For this review, take the finished solid that the model builds, in its own axes (mm). A direction names the side the tool comes from. Round coordinates to 2 decimals unless told otherwise and drop trailing zeros. Loops run counter-clockwise (first coordinate to the right, second up) from the corner with the lowest first, then second, coordinate; pieces in that order, holes last. Notation, with made-up numbers: (41, -8) -> (92, -8) arc R24 ccw to (92, 2) -> close; hole circle Ø2 at (65, 54). An arc over 180 degrees is marked (long way). Write each question's results on one line, items separated by ' | '.
```python
from build123d import *
from OCP.BRepFilletAPI import BRepFilletAPI_MakeChamfer

# Parameters (mm, degrees)
SKETCH1_W           = 60
SKETCH1_H           = 27
BOSS_EXTRUDE1_DEPTH = 6
SKETCH2_R           = 13.5
SKETCH2_R_2         = 8.5
BOSS_EXTRUDE2_DEPTH = 30
SKETCH3_W           = 60
SKETCH3_H           = 5
BOSS_EXTRUDE3_DEPTH = 30
CHAMFER1_SIZE       = 30
CHAMFER1_SIZE2      = 19.5
SKETCH5_R           = 2.5
CUT_EXTRUDE1_DEPTH  = 30
CHAMFER3_SIZE       = 1


with BuildPart() as part:
    # Sketch1 → Boss-Extrude1 (new body)
    with BuildSketch(Plane(origin=(0, 0, 0), x_dir=(1, 0, 0), z_dir=(0, 1, 0))):
        with Locations((-76.040322581, 2.721774194)):
            Rectangle(SKETCH1_W, SKETCH1_H)
    extrude(amount=BOSS_EXTRUDE1_DEPTH)

    # Sketch2 → Boss-Extrude2 (add)
    with BuildSketch(Plane(origin=(0, 6, 0), x_dir=(1, 0, 0), z_dir=(0, 1, 0))):
        with Locations(Location((-76.040322581, 2.721774194, 0), (0, 0, 270))):
            Circle(SKETCH2_R)
        with Locations(Location((-76.040322581, 2.721774194, 0), (0, 0, 270))):
            Circle(SKETCH2_R_2, mode=Mode.SUBTRACT)
    extrude(amount=BOSS_EXTRUDE2_DEPTH)

    # Sketch3 → Boss-Extrude3 (add)
    with BuildSketch(Plane(origin=(0, 6, 0), x_dir=(1, 0, 0), z_dir=(0, 1, 0))):
        with Locations((-76.040322581, 13.721774194)):
            Rectangle(SKETCH3_W, SKETCH3_H)
        with Locations((-76.040322581, -8.278225806)):
            Rectangle(SKETCH3_W, SKETCH3_H)
    extrude(amount=BOSS_EXTRUDE3_DEPTH)

    # Chamfer1: one chamfer whose edges measure the first distance from different faces: ONE call of the kernel's chamfer builder (chamfer() names one face for all edges)
    chamfer1_edges_1 = [part.edges().sort_by_distance(p)[0] for p in [
        (-46.040322581, 36, 8.278225806),
        (-46.040322581, 36, -13.721774194),
    ]]
    chamfer1_side_1 = [part.faces().sort_by_distance(p)[0] for p in [
        (-46.040322581, 18, -15.771774194),
    ]]
    chamfer1_edges_2 = [part.edges().sort_by_distance(p)[0] for p in [
        (-106.040322581, 36, 8.278225806),
        (-106.040322581, 36, -13.721774194),
    ]]
    chamfer1_side_2 = [part.faces().sort_by_distance(p)[0] for p in [
        (-106.040322581, 18, 10.328225806),
    ]]
    chamfer1 = BRepFilletAPI_MakeChamfer(part.part.solid().wrapped)
    for e in chamfer1_edges_1:
        chamfer1.Add(CHAMFER1_SIZE, CHAMFER1_SIZE2, e.wrapped, chamfer1_side_1[0].wrapped)  # the first distance lies on this face
    for e in chamfer1_edges_2:
        chamfer1.Add(CHAMFER1_SIZE, CHAMFER1_SIZE2, e.wrapped, chamfer1_side_2[0].wrapped)  # the first distance lies on this face
    add(Compound.cast(chamfer1.Shape()), mode=Mode.REPLACE)

    # Sketch5 → Cut-Extrude1 (cut)
    with BuildSketch(Plane(origin=(0, 6, 0), x_dir=(1, 0, 0), z_dir=(0, 1, 0))):
        with Locations(Location((-96.284366821, 2.721774194, 0), (0, 0, 270))):
            Circle(SKETCH5_R)
        with Locations(Location((-55.79627834, 2.721774194, 0), (0, 0, 270))):
            Circle(SKETCH5_R)
    extrude(amount=-CUT_EXTRUDE1_DEPTH, mode=Mode.SUBTRACT)

    # Chamfer3
    chamfer3_edges = [part.edges().sort_by_distance(p)[0] for p in [
        (-76.040322581, 36, -11.221774194),
    ]]
    chamfer(chamfer3_edges, length=CHAMFER3_SIZE)


solid = part.part
```
1. Consider section B-B (y = 7.5). State the section outline as (x, z) points.
Values found:
outline: (-105.07, -16.22) -> (-47.02, -16.22) -> (-47.02, -11.22) -> (-65.55, -11.22) arc R13.5 ccw to (-65.55, 5.78) -> (-47.02, 5.78) -> (-47.02, 10.78) -> (-105.07, 10.78) -> (-105.07, 5.78) -> (-86.53, 5.78) arc R13.5 ccw to (-86.53, -11.22) -> (-105.07, -11.22) -> close; hole circle Ø17 at (-76.04, -2.72)
2. For pin 1 (15.5 mm diameter, centred on x = -76.04, z = -2.72, fed in from +Y); pin 2 (5 mm diameter, centred on y = 30.5, z = 5, fed in from +X); pin 3 (1.5 mm diameter, centred on y = 30.5, z = -10, fed in from +X), all flat-tipped, find the tip position at first contact; note any pin that passes through.
Values found:
pin 1: stops at y = 6 | pin 2: stops at x = -60.42 | pin 3: stops at x = -64.22
3. To check wall thickness, follow probe 1 along Z at (x, y) = (-76.5, 28); probe 2 along Z at (x, y) = (-64.5, 6.5); probe 3 along X at (y, z) = (23.5, 4). State the ranges of each line that lie inside material, in increasing order.
Values found:
probe 1: z = -16.22 to -11.21, 5.77 to 10.78 | probe 2: z = -16.22 to -11.22, -9.73 to 4.28, 5.78 to 10.78 | probe 3: x = -87.75 to -81.24, -70.84 to -64.33
4. Tool access review of faces 1 (the face through (-76, 6, -3)), 2 (the face through (-54, 6, -5)), 3 (the face through (-99, 6, -5)), 4 (the face through (-106.04, 3, -3)), 5 (the face through (-76, 14, -16.222)): name each direction out of +Z, -Z, +X, -X, +Y, -Y from which nothing blocks a thin tool from reaching the whole face with its end or side.
Values found:
face 1: +Y | face 2: +X, +Y | face 3: -X, +Y | face 4: +Z, -Z, -X, +Y, -Y | face 5: -Z, +X, -X, +Y, -Y
5. Consider section A-A (x = -98). State the section outline as (y, z) points.
Values found:
outline: (0, -16.22) -> (18.37, -16.22) -> (18.37, -11.22) -> (6, -11.22) -> (6, -4.54) -> (0, -4.54) -> close; (0, -0.9) -> (6, -0.9) -> (6, 5.78) -> (18.37, 5.78) -> (18.37, 10.78) -> (0, 10.78) -> close
6. Consider section C-C (x = -59). State the section outline as (y, z) points, plus the area to 3 significant figures.
Values found:
outline: (0, -16.22) -> (25.94, -16.22) -> (25.94, -11.22) -> (6, -11.22) -> (6, 5.78) -> (25.94, 5.78) -> (25.94, 10.78) -> (0, 10.78) -> close | area: 361 mm2
7. Consider section D-D (z = 8.5). State the section outline as (x, y) points.
Values found:
outline: (-106.04, 0) -> (-46.04, 0) -> (-46.04, 6) -> (-65.54, 36) -> (-86.54, 36) -> (-106.04, 6) -> close
